Could you check a few things on this model? Use its own coordinates, in mm. A direction names the side the tool comes from. Give positions to 0.01 mm unless a question says otherwise; leave off trailing zeros. Write each loop counter-clockwise with the first axis right and the second up, starting at its lowest first coordinate (ties: lowest second). Pieces come first, ordered by that corner, then holes. Notation, with made-up numbers: (-18.75, 63.5) - (23.25, 63.5) arc R21 cw to (23.25, 75.5) - close; hole circle Ø4 at (66, 47.5). An arc over 180 degrees is marked (long way). Answer in a Markdown table with one row per item.
from build123d import *

# Parameters (mm, degrees)
SKETCH1_R           = 7.5
BOSS_EXTRUDE1_DEPTH = 25
CUT_EXTRUDE1_DEPTH  = 34
SKETCH3_W           = 45
SKETCH3_H           = 19
CUT_EXTRUDE2_DEPTH  = 62
SKETCH4_R           = 1.5
CUT_EXTRUDE3_DEPTH  = 62


with BuildPart() as part:
    # Sketch1 → Boss-Extrude1 (new, symmetric)
    with BuildSketch(Plane(origin=(0, 0, 0), x_dir=(0, 0, -1), z_dir=(1, 0, 0))):
        Polygon((-32.5, -10.5), (-43, -10.5), (-43, 12.5), (43, 12.5), (43, -10.5), align=None)
        with Locations((-32.5, 0)):
            Circle(SKETCH1_R, mode=Mode.SUBTRACT)
        with Locations(Location((32.5, 0, 0), (0, 0, 180))):
            Circle(SKETCH1_R, mode=Mode.SUBTRACT)
    extrude(amount=BOSS_EXTRUDE1_DEPTH, both=True)

    # Sketch2 → Cut-Extrude1 (cut)
    with BuildSketch(Plane.XZ.offset(10.5)):
        Polygon((14, -13.850798543), (-18, -13.850798543), (-18, 2.304286058), (-14, 2.304286058), (-14, 18.660685655), (14, 18.660685655), align=None)
    extrude(amount=-CUT_EXTRUDE1_DEPTH, mode=Mode.SUBTRACT)

    # Sketch3 → Cut-Extrude2 (cut)
    with BuildSketch(Plane.ZY.offset(25)):
        with Locations((0, -1)):
            Rectangle(SKETCH3_W, SKETCH3_H)
    extrude(amount=-CUT_EXTRUDE2_DEPTH, mode=Mode.SUBTRACT)

    # Sketch4 → Cut-Extrude3 (cut)
    with BuildSketch(Plane.XZ.offset(-8.5)):
        with Locations(Location((-21, -6.058605683, 0), (0, 0, 270))):
            Circle(SKETCH4_R)
        with Locations(Location((19, -6.058605683, 0), (0, 0, 270))):
            Circle(SKETCH4_R)
    extrude(amount=-CUT_EXTRUDE3_DEPTH, mode=Mode.SUBTRACT)


solid = part.part
1) Imagine slicing it at D-D (x = 3.5). List the corners of the cut face in (y, z) for me, then the cut area to 3 significant figures.
Check values:
| item | result |
|---|---|
| outline | (-10.5, -43) - (12.5, -43) - (12.5, -13.85) - (8.5, -13.85) - (8.5, -22.5) - (-10.5, -22.5) - close; (-10.5, 22.5) - (8.5, 22.5) - (8.5, 18.66) - (12.5, 18.66) - (12.5, 43) - (-10.5, 43) - close; hole circle Ø15 at (0, -32.5); hole circle Ø15 at (0, 32.5) |
| area | 640 mm2 |
2) We'd pull the mould along Z, two halves only. Please class faces 1 (the face through (-25, 10, 0)), 2 (the face through (0, 1, -43)), 3 (the face through (14, 10, 3)): +Z half, -Z half, draft (parallel to the pull), parting line (faces both ways), or undercut.
Check values:
| item | result |
|---|---|
| face 1 | draft |
| face 2 | -Z half |
| face 3 | undercut |
3) Imagine slicing it at B-B (z = -1). List the corners of the cut face in (x, y) for me.
Check values:
| item | result |
|---|---|
| outline | (-25, 8.5) - (-18, 8.5) - (-18, 12.5) - (-25, 12.5) - close; (14, 8.5) - (25, 8.5) - (25, 12.5) - (14, 12.5) - close |
4) Imagine slicing it at A-A (x = -21). List the corners of the cut face in (y, z) for me.
Check values:
| item | result |
|---|---|
| outline | (-10.5, -43) - (12.5, -43) - (12.5, -7.56) - (8.5, -7.56) - (8.5, -22.5) - (-10.5, -22.5) - close; (-10.5, 22.5) - (8.5, 22.5) - (8.5, -4.56) - (12.5, -4.56) - (12.5, 43) - (-10.5, 43) - close; hole circle Ø15 at (0, -32.5); hole circle Ø15 at (0, 32.5) |
5) Imagine slicing it at C-C (y = 4.25). List the corners of the cut face in (x, z) for me, then the cut area to 3 significant figures.
Check values:
| item | result |
|---|---|
| outline | (-25, -43) - (25, -43) - (25, -38.68) - (-25, -38.68) - close; (-25, -26.32) - (25, -26.32) - (25, -22.5) - (-25, -22.5) - close; (-25, 22.5) - (25, 22.5) - (25, 26.32) - (-25, 26.32) - close; (-25, 38.68) - (25, 38.68) - (25, 43) - (-25, 43) - close |
| area | 814 mm2 |
6) If I drill on line 1 (X direction, y = 9, z = 11); line 2 (Z direction, x = -1.5, y = 7.75); line 3 (Y direction, x = 14, z = -32.5), over which ranges is the centre line in solid material (lowest first)?
Check values:
| item | result |
|---|---|
| line 1 | x = -25 to -14, 14 to 25 |
| line 2 | z = -43 to -22.5, 22.5 to 43 |
| line 3 | y = -10.5 to -7.5, 7.5 to 12.5 |
7) On a 3-axis mill with a long thin cutter (end or side, diameter ignored), from which of +Z, -Z, +X, -X, +Y, -Y can I reach the whole of each face in a straight line? I mean faces 4 (the face through (0, -10.5, -33)), 5 (the face through (0, 8.5, -15)), 6 (the face through (-16, 10, 2.304)). Say none if no direction works.
Check values:
| item | result |
|---|---|
| face 4 | +Z, -Z, +X, -X, -Y |
| face 5 | +X, -X, -Y |
| face 6 | +Y, -Y |
